Geometry: see drawing. Coordinates: mm, zero at the bounding-box minimum. Round coordinates to 2 decimals unless told otherwise and drop trailing zeros. Loops run counter-clockwise (first coordinate to the right, second up) from the corner with the lowest first, then second, coordinate; pieces in that order, holes last. Notation, with made-up numbers: (75.25, 52) - (129.25, 52) arc R20 cw to (129.25, 60) - close; hole circle Ø5 at (29, 69). An arc over 180 degrees is marked (long way). Use CSV: the item, a comma, the result in double quotes. Start each with the question number.
1. Material intervals for probe 1 along X at (y, z) = (29.5, 52.5); probe 2 along Y at (x, z) = (28, 29); probe 3 along Z at (x, y) = (28.5, 31), sorted ascending. Write a range as from..to.
2. Cut plane A-A (x = 28.5). Return loops of the section in (y, z).
3. Cut plane C-C (z = 54.5). Return loops of the section in (x, y), and give its area (3 significant figures).
4. Pin query (flat end, axial travel): P1, Ø4, axis at x = 18.5, z = 19.5, coming from the +Y side; P2, Ø3, axis at y = 6, z = 39.5, coming from the +X side; P3, Ø2, axis at x = 48, z = 17.5, coming from the +Y side. Return the tip coordinate at first contact, or that it passes through.
5. Pull-direction query (X, two-part tool) for the marked faces 1, 2 and 3; classes: +X half, -X half, draft (parallel to the pull), parting line (faces both ways), or undercut.
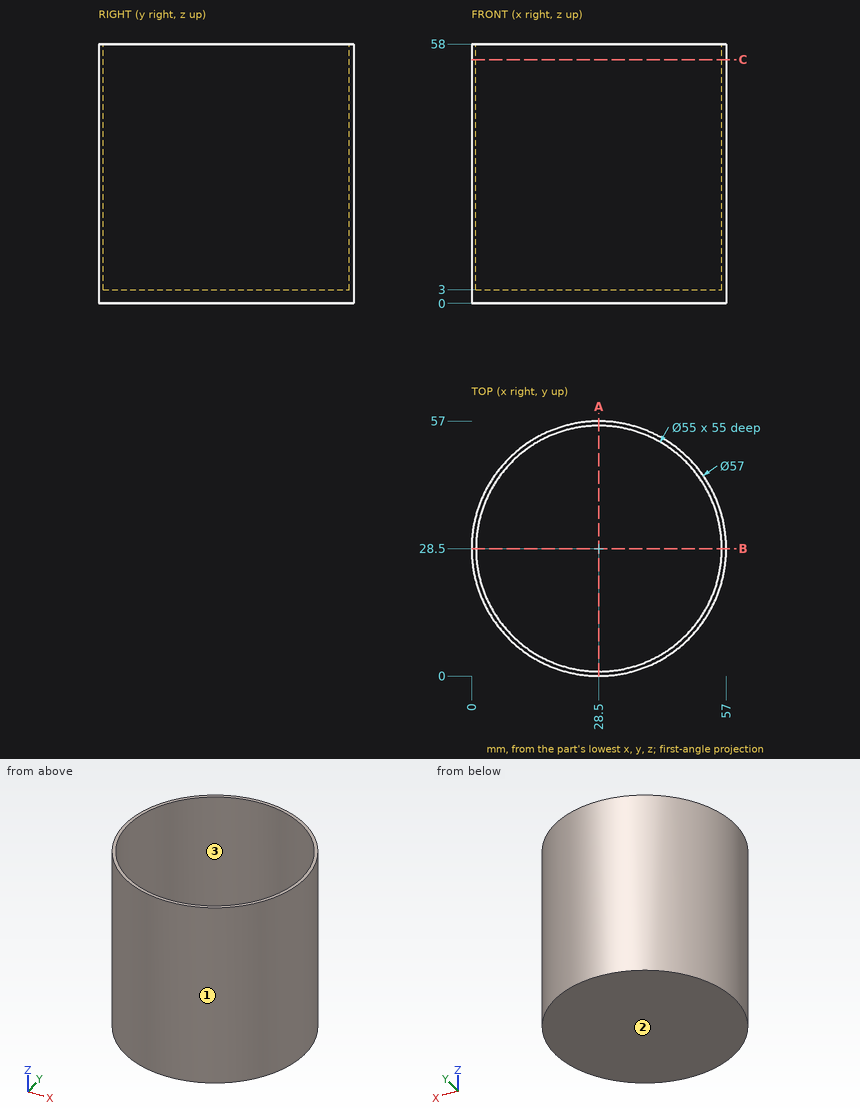
Established:
1,probe 1,"x = 0.02..1.02, 55.98..56.98"
1,probe 2,"y = 0..1, 56..57"
1,probe 3,"z = 0..3"
2,outline,"(0, 0) - (57, 0) - (57, 58) - (56, 58) - (56, 3) - (1, 3) - (1, 58) - (0, 58) - close"
3,outline,"circle Ø57 at (28.5, 28.5); hole circle Ø55 at (28.5, 28.5)"
3,area,"176 mm2"
4,P1,"stops at y = 55.85"
4,P2,"stops at x = 47.77"
4,P3,"stops at y = 50.18"
5,face 1,"parting line"
5,face 2,"draft"
5,face 3,"undercut"
